```python
from build123d import *

# Parameters (mm, degrees)
SKIZZE1_R                          = 4.5
SKIZZE1_R_2                        = 1.65
AUFSATZ_LINEAR_AUSTRAGEN1_DEPTH    = 8
SKIZZE2_R                          = 4.5
SKIZZE2_R_2                        = 1.65
AUFSATZ_LINEAR_AUSTRAGEN2_DEPTH    = 3
FASE1_SIZE                         = 2
FASE1_SIZE2                        = 5.494954839
SKIZZE3_R                          = 3
SCHNITT_LINEAR_AUSTRAGEN1_DEPTH    = 3
K_RPER_VERSCHIEBEN_KOPIEREN1_ANGLE = 90


with BuildPart() as part:
    # Skizze1 → Aufsatz-Linear austragen1 (new body)
    with BuildSketch(Plane(origin=(0, 0, 0), x_dir=(1, 0, 0), z_dir=(0, 1, 0))):
        Polygon((286, 0), (286, -6.26), (276.8, -6.26), (276.8, -15.9), (286, -15.9), (286, -19.6), (0, -19.6), (0, -15.9), (9.2, -15.9), (9.2, -6.26), (0, -6.26), (0, 0), align=None)
        with Locations(Location((260, -9.8, 0), (0, 0, 270))):
            Circle(SKIZZE1_R, mode=Mode.SUBTRACT)
        with Locations(Location((26, -9.8, 0), (0, 0, 270))):
            Circle(SKIZZE1_R, mode=Mode.SUBTRACT)
        with Locations(Location((14, -5.8, 0), (0, 0, 270))):
            Circle(SKIZZE1_R_2, mode=Mode.SUBTRACT)
        with Locations(Location((78.5, -13.8, 0), (0, 0, 270))):
            Circle(SKIZZE1_R_2, mode=Mode.SUBTRACT)
        with Locations(Location((121.5, -5.8, 0), (0, 0, 270))):
            Circle(SKIZZE1_R_2, mode=Mode.SUBTRACT)
        with Locations(Location((164.5, -13.8, 0), (0, 0, 270))):
            Circle(SKIZZE1_R_2, mode=Mode.SUBTRACT)
        with Locations(Location((207.5, -5.8, 0), (0, 0, 270))):
            Circle(SKIZZE1_R_2, mode=Mode.SUBTRACT)
        with Locations(Location((272, -13.8, 0), (0, 0, 270))):
            Circle(SKIZZE1_R_2, mode=Mode.SUBTRACT)
        Polygon((200.330127019, -2.3), (204.660254038, -9.8), (200.330127019, -17.3), (171.669872981, -17.3), (167.339745962, -9.8), (171.669872981, -2.3), align=None, mode=Mode.SUBTRACT)
        Polygon((243.330127019, -2.3), (247.660254038, -9.8), (243.330127019, -17.3), (214.669872981, -17.3), (210.339745962, -9.8), (214.669872981, -2.3), align=None, mode=Mode.SUBTRACT)
        Polygon((81.339745962, -9.8), (85.669872981, -2.3), (114.330127019, -2.3), (118.660254038, -9.8), (114.330127019, -17.3), (85.669872981, -17.3), align=None, mode=Mode.SUBTRACT)
        Polygon((38.339745962, -9.8), (42.669872981, -2.3), (71.330127019, -2.3), (75.660254038, -9.8), (71.330127019, -17.3), (42.669872981, -17.3), align=None, mode=Mode.SUBTRACT)
        Polygon((128.669872981, -2.3), (157.330127019, -2.3), (161.660254038, -9.8), (157.330127019, -17.3), (128.669872981, -17.3), (124.339745962, -9.8), align=None, mode=Mode.SUBTRACT)
    extrude(amount=AUFSATZ_LINEAR_AUSTRAGEN1_DEPTH)

    # Skizze2 → Aufsatz-Linear austragen2 (add)
    with BuildSketch(Plane(origin=(0, 8, 0), x_dir=(1, 0, 0), z_dir=(0, 1, 0))):
        Polygon((0, -19.6), (286, -19.6), (286, -15.9), (276.8, -15.9), (276.8, -6.26), (286, -6.26), (286, 0), (0, 0), (0, -6.26), (9.2, -6.26), (9.2, -15.9), (0, -15.9), align=None)
        with Locations(Location((260, -9.8, 0), (0, 0, 270))):
            Circle(SKIZZE2_R, mode=Mode.SUBTRACT)
        with Locations(Location((26, -9.8, 0), (0, 0, 270))):
            Circle(SKIZZE2_R, mode=Mode.SUBTRACT)
        with Locations(Location((272, -13.8, 0), (0, 0, 270))):
            Circle(SKIZZE2_R_2, mode=Mode.SUBTRACT)
        with Locations(Location((207.5, -5.8, 0), (0, 0, 270))):
            Circle(SKIZZE2_R_2, mode=Mode.SUBTRACT)
        with Locations(Location((164.5, -13.8, 0), (0, 0, 270))):
            Circle(SKIZZE2_R_2, mode=Mode.SUBTRACT)
        with Locations(Location((78.5, -13.8, 0), (0, 0, 270))):
            Circle(SKIZZE2_R_2, mode=Mode.SUBTRACT)
        with Locations(Location((121.5, -5.8, 0), (0, 0, 270))):
            Circle(SKIZZE2_R_2, mode=Mode.SUBTRACT)
        with Locations(Location((14, -5.8, 0), (0, 0, 270))):
            Circle(SKIZZE2_R_2, mode=Mode.SUBTRACT)
    extrude(amount=AUFSATZ_LINEAR_AUSTRAGEN2_DEPTH)

    # Fase1
    fase1_edges = [part.edges().sort_by_distance(p)[0] for p in [
        (143, 11, 19.6),
        (143, 11, 0),
    ]]
    fase1_side = [part.faces().sort_by_distance(p)[0] for p in [
        (143, 11, 9.756751336),
    ]]
    chamfer(fase1_edges, length=FASE1_SIZE, length2=FASE1_SIZE2, reference=fase1_side[0])

    # Skizze3 → Schnitt-Linear austragen1 (cut)
    with BuildSketch(Plane(origin=(0, 11, 0), x_dir=(1, 0, 0), z_dir=(0, 1, 0))):
        with Locations(Location((14, -5.8, 0), (0, 0, 270))):
            Circle(SKIZZE3_R)
        with Locations(Location((78.5, -13.8, 0), (0, 0, 270))):
            Circle(SKIZZE3_R)
        with Locations(Location((121.5, -5.8, 0), (0, 0, 270))):
            Circle(SKIZZE3_R)
        with Locations(Location((164.5, -13.8, 0), (0, 0, 270))):
            Circle(SKIZZE3_R)
        with Locations(Location((207.5, -5.8, 0), (0, 0, 270))):
            Circle(SKIZZE3_R)
        with Locations(Location((272, -13.8, 0), (0, 0, 270))):
            Circle(SKIZZE3_R)
    extrude(amount=-SCHNITT_LINEAR_AUSTRAGEN1_DEPTH, mode=Mode.SUBTRACT)


with BuildPart() as part_1:
    # Körper-Verschieben/Kopieren1: moved
    add(part.part.rotate(Axis((0, 5.5, 9.8), (1, 0, 0)), K_RPER_VERSCHIEBEN_KOPIEREN1_ANGLE))


solid = part_1.part
```
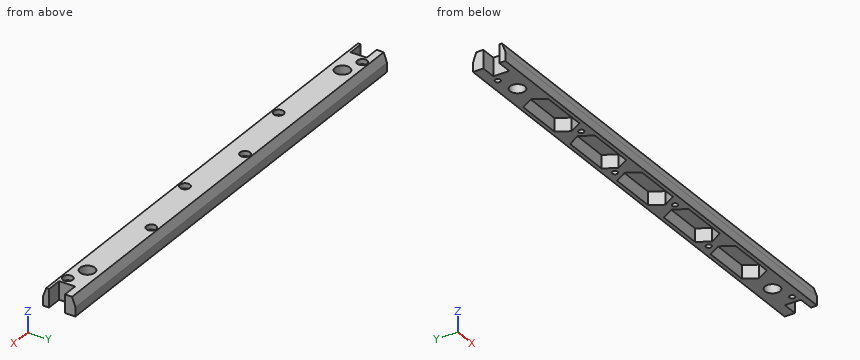
Model file for the job. Use its own axes, mm. Give positions to 0.01 mm unless a question says otherwise; leave off trailing zeros. Order: outer loops, then holes, each group sorted by start corner. A loop starts at its lowest first (then second) coordinate and runs counter-clockwise, first axis right, second up.
1) Saw through at B-B, the plane x = 224.5. Write the cut outline in (y, z), then the cut area to 3 significant figures.
2) Pin check, flat tips, straight feed: pin 1 (4.5 mm diameter, centred on x = 53.5, y = 2.5, fed in from -Z); pin 2 (3 mm diameter, centred on x = 273, y = 2.5, fed in from +Z). Stop position of each tip, or through.
3) Saw through at A-A, the plane x = 26. Write the cut outline in (y, z), then the cut area to 3 significant figures.
4) Wall check: probe 1 along Y at (x, z) = (132.5, 5.5); probe 2 along X at (y, z) = (10.5, 13.5); probe 3 along Y at (x, z) = (121.5, 6.5). Give the ranges that are in metal, low to high.
Computed:
1. outline: (-4.3, 4.3) - (-2, 4.3) - (-2, 12.3) - (13, 12.3) - (13, 4.3) - (15.3, 4.3) - (15.3, 9.81) - (13.3, 15.3) - (-2.3, 15.3) - (-4.3, 9.81) - close
1. area: 84.6 mm2
2. pin 1: stops at z = 12.3
2. pin 2: stops at z = 12.3
3. outline: (-4.3, 4.3) - (1, 4.3) - (1, 15.3) - (-2.3, 15.3) - (-4.3, 9.81) - close; (10, 4.3) - (15.3, 4.3) - (15.3, 9.81) - (13.3, 15.3) - (10, 15.3) - close
3. area: 106 mm2
4. probe 1: y = -4.3 to -2, 13 to 15.3
4. probe 2: x = 0 to 11.17, 16.83 to 118.67, 124.33 to 204.67, 210.33 to 286
4. probe 3: y = -4.3 to 7.85, 11.15 to 15.3
